The model under review builds one solid part; all positions refer to its coordinate system, in mm. Coordinates: 2 decimals unless noted, no trailing zeros. Write each loop counter-clockwise with the first axis right and the second up, starting at its lowest first coordinate (ties: lowest second). Pieces come first, ordered by that corner, then holes. Notation, with made-up numbers: (14, 54) - (27, 54) arc R27 ccw to (27, 74) - close; hole circle Ø1 at (59, 51). An arc over 180 degrees is marked (long way). Use one line per item in the form item = value. Start each with the question number.
Autodesk Inventor part; units mm, degrees
ref_plane "YZ Plane" through (0, 0, 0) normal (1, 0, 0) x (0, 1, 0)
ref_plane "XZ Plane" through (0, 0, 0) normal (0, 1, 0) x (-1, 0, 0)
ref_plane "XY Plane" through (0, 0, 0) normal (0, 0, 1) x (1, 0, 0)
sketch "Sketch1" plane through (0, 0, 0) normal (1, 0, 0) x (0, 1, 0)
  line L0 (0, 0) -> (38.1, 0)
  line L1 (38.1, 0) -> (38.1, -19.05)
  line L2 (38.1, -19.05) -> (0, -19.05)
  line L3 (0, -19.05) -> (0, 0)
  line L4 (0, 0) -> (0, -0.7937)
  line L5 (0, -0.7937) -> (12.7, -0.7937)
  line L6 (12.7, -0.7937) -> (38.1, -12.638) construction
  line L7 (38.1, -12.638) -> (38.1, 0)
  line L8 (0, 0) -> (0, -0.7937)
  line L9 (12.7, -0.7937) -> (38.1, -12.638)
  line L10 (12.7, -0.7937) -> (40.7258, -0.7937) construction
  line L11 (0, -19.05) -> (5.8372, -13.2128)
  line L12 (0, -19.05) -> (8.255, -19.05) construction
  point P0 (8.255, 8.255)
  dimension "partH" = 38.1
  dimension "partR" = 19.05
  dimension "tubeID" = 0.7937
  dimension "straightDepth" = 12.7
  dimension "funnelTaperAngle" = 155
  dimension "taperAngle" = 25
  dimension "d15" = 8.255
  dimension "d16" = 45
revolve "Revolution1" add sketch "Sketch1" angle 360 about axis through (0, 0, 0) along (0, 1, 0) contours L5 L9 L1 L2 L3
sketch "Sketch2" plane through (0, 0, 0) normal (0, -1, 0) x (1, 0, 0)
  point P0 (0, 0)
  point P1 (0, 0)
hole "Hole1" at (0, 0, 0) direction (0, 1, 0) diameter 5.3594 depth 9.525 tip angle 118
sketch "Sketch3" plane through (0, 0, 0) normal (0, -1, 0) x (1, 0, 0)
  circle A0 centre (0, 0) radius 0.7937
  line L0 (0, 0) -> (0, -19.05)
  circle A1 centre (0, 0) radius 19.05
ref_plane "Work Plane1" through (0, 0, 0) normal (-1, 0, 0) x (0, 0, -1)
sketch "Sketch4" plane through (0, 0, 0) normal (-1, 0, 0) x (0, 0, -1)
  line L0 (19.05, 0) -> (-19.05, 0)
  line L1 (-19.05, 0) -> (-11.8658, -7.1842)
  line L2 (-19.05, 0) -> (-8.89, 0) construction
  line L3 (19.05, 0) -> (11.8658, -7.1842)
  line L4 (19.05, 0) -> (29.21, 0) construction
  point P0 (0, 0)
  dimension "d18" = 10.16
  dimension "d19" = 45
  dimension "d20" = 10.16
  dimension "d21" = 135
properties part number "ptfe_catch_no_mount"
1. Take a section at D-D (y = 30.5). State the section outline as (x, z) points.
2. Take a section at B-B (z = 0). State the section outline as (x, y) points (3 decimals).
3. For L1, parallel to Z at x = 0, y = 12.2; L2, parallel to X at y = 4, z = 0, list the stretches that pass through material, from the lowest coordinate up.
4. For P1, Ø10, axis at y = 23.5, z = 3, coming from the -X side; P2, Ø1, axis at x = 0, z = 0, coming from the -Y side; P3, Ø2, axis at y = 31, z = -3, coming from the +X side; P4, Ø10, axis at y = 31, z = -1.5, coming from the +X side, all flat-tipped, find the tip position at first contact; note any pin that passes through.
5. Take a section at A-A (x = 0). State the section outline as (y, z) points (3 decimals), plus the area to 3 significant figures.
6. Take a section at C-C (y = 5). State the section outline as (x, z) points, plus the area to 3 significant figures.
7. The part is to be moulded in two halves that separate along X. For faces 1 (the cylindrical face through (-11.59, 18.78, 15.12)), 2 (the cylindrical face through (-0.118, 4.829, 2.677)), 3 (the flat face through (4, 38.1, -12.4)), say which applies: released by +X, released by -X, zero draft, split by the parting line, or undercut.
Returned:
q1.outline = circle Ø38.1 at (0, 0); hole circle Ø18.19 at (0, 0)
q2.outline = (-19.05, 0) - (-2.68, 0) - (-2.68, 9.525) - (-0.794, 10.658) - (-0.794, 12.7) - (-12.638, 38.1) - (-19.05, 38.1) - close; (0.794, 10.658) - (2.68, 9.525) - (2.68, 0) - (19.05, 0) - (19.05, 38.1) - (12.638, 38.1) - (0.794, 12.7) - close
q3.L1 = -19.05 to -0.79, 0.79 to 19.05
q3.L2 = -19.05 to -2.68, 2.68 to 19.05
q4.P1 = -19.05
q4.P2 = through
q4.P3 = 18.94
q4.P4 = 19.05
q5.outline = (0, -19.05) - (38.1, -19.05) - (38.1, -12.638) - (12.7, -0.794) - (10.658, -0.794) - (9.525, -2.68) - (0, -2.68) - close; (0, 2.68) - (9.525, 2.68) - (10.658, 0.794) - (12.7, 0.794) - (38.1, 12.638) - (38.1, 19.05) - (0, 19.05) - close
q5.area = 1,050 mm²
q6.outline = circle Ø38.1 at (0, 0); hole circle Ø5.36 at (0, 0)
q6.area = 1,120 mm²
q7.face_1 = split by the parting line
q7.face_2 = undercut
q7.face_3 = zero draft
